Can you work these out from the model? Positions are in its coordinate system, mm. Face numbers are marked on the shaded views. A direction names the side the tool comes from. Coordinates: 2 decimals unless noted, no trailing zeros. Order: outer loops, then holes, each group sorted by start corner. A loop starts at its lowest first (then second) coordinate and runs counter-clockwise, first axis right, second up.
```python
from build123d import *

# Parameters (mm, degrees)
F0_R     = 9.806931969
F0_R_2   = 2.6876925043
F1_DEPTH = 1.905
F2_DEPTH = 4.3688


# Not quite as in the source:
# - a fillet or chamfer that OpenCascade refuses, or shapes differently, is made with other operations: its cross-section is extruded or revolved along the edge and cut away or added


with BuildPart() as f1:
    # F0 (on Top) → F1 (new body)
    with BuildSketch(Plane.XY):
        Circle(F0_R)
        Circle(F0_R_2, mode=Mode.SUBTRACT)
        Circle(F0_R_2)
    extrude(amount=F1_DEPTH)

    # F0 (on Top) → F2 (join)
    with BuildSketch(Plane.XY):
        Circle(F0_R_2)
    extrude(amount=-F2_DEPTH)

    # F3: fillet of radius 5.08 on 1 edges, made by hand

    # F3_s1 → F3_t2 (revolve, cut)
    with BuildSketch(Plane.XZ):
        with BuildLine():
            ThreePointArc((9.806931969, 0), (8.0410627657, 1.4040501198), (5.8413582401, 1.905))
            Line((5.8413582401, 1.905), (9.806931969, 1.905))
            Line((9.806931969, 1.905), (9.806931969, 0))
        make_face()
    revolve(axis=Axis((0, 0, 1.905), (0, 0, 1)), mode=Mode.SUBTRACT)


solid = f1.part
```
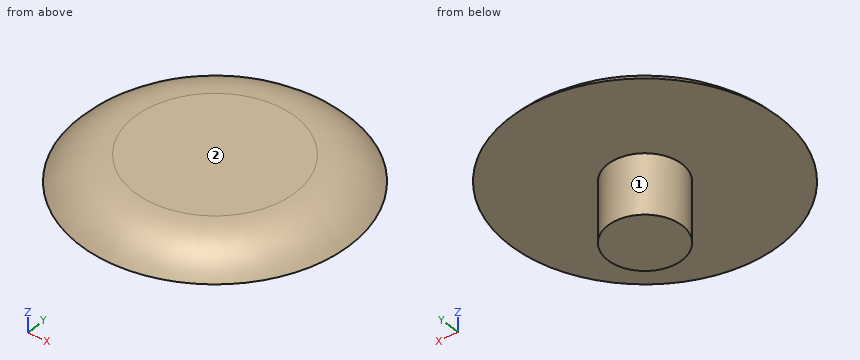
1. Imagine slicing it at D-D on z = 1. Please give me the cut outline in (x, y).
Completed:
outline: circle Ø17.47 at (0, 0)
2. Imagine slicing it at C-C on z = -3.5. Please give me the cut outline in (x, y), then the cut area to 3 significant figures.
Completed:
outline: circle Ø5.38 at (0, 0)
area: 22.7 mm2
3. I'm going to push flat-ended pins straight in: pin 1 (1.5 mm diameter, centred on x = -1.5, z = -0.5, fed in from -Y); pin 2 (2 mm diameter, centred on x = -5.5, z = -3.5, fed in from +Y); pin 3 (4 mm diameter, centred on x = -1, y = 6.5, fed in from -Z). Where does each tip first touch, or does it pass through?
Completed:
pin 1: stops at y = -9.76
pin 2: passes through
pin 3: stops at z = 0
4. On a 3-axis mill with a long thin cutter (end or side, diameter ignored), from which of +Z, -Z, +X, -X, +Y, -Y can I reach the whole of each face in a straight line? I mean the marked faces 1 and 2. Say none if no direction works.
Completed:
face 1: -Z
face 2: +Z, +X, -X, +Y, -Y
5. Please list where these lines run through material, in increasing order: probe 1 along Z at (x, y) = (4.25, -3) (3 decimals); probe 2 along X at (y, z) = (5.5, 1); probe 3 along Y at (x, z) = (-3.75, 0.5).
Completed:
probe 1: z = 0 to 1.905
probe 2: x = -6.79 to 6.79
probe 3: y = -8.56 to 8.56
6. Imagine slicing it at A-A on x = 0. Please give me the cut outline in (y, z) (3 decimals), then the cut area to 3 significant figures.
Completed:
outline: (-9.807, 0) - (-2.688, 0) - (-2.688, -4.369) - (2.688, -4.369) - (2.688, 0) - (9.807, 0) arc R5.08 ccw to (5.841, 1.905) - (-5.841, 1.905) arc R5.08 ccw to start
area: 56.3 mm2
